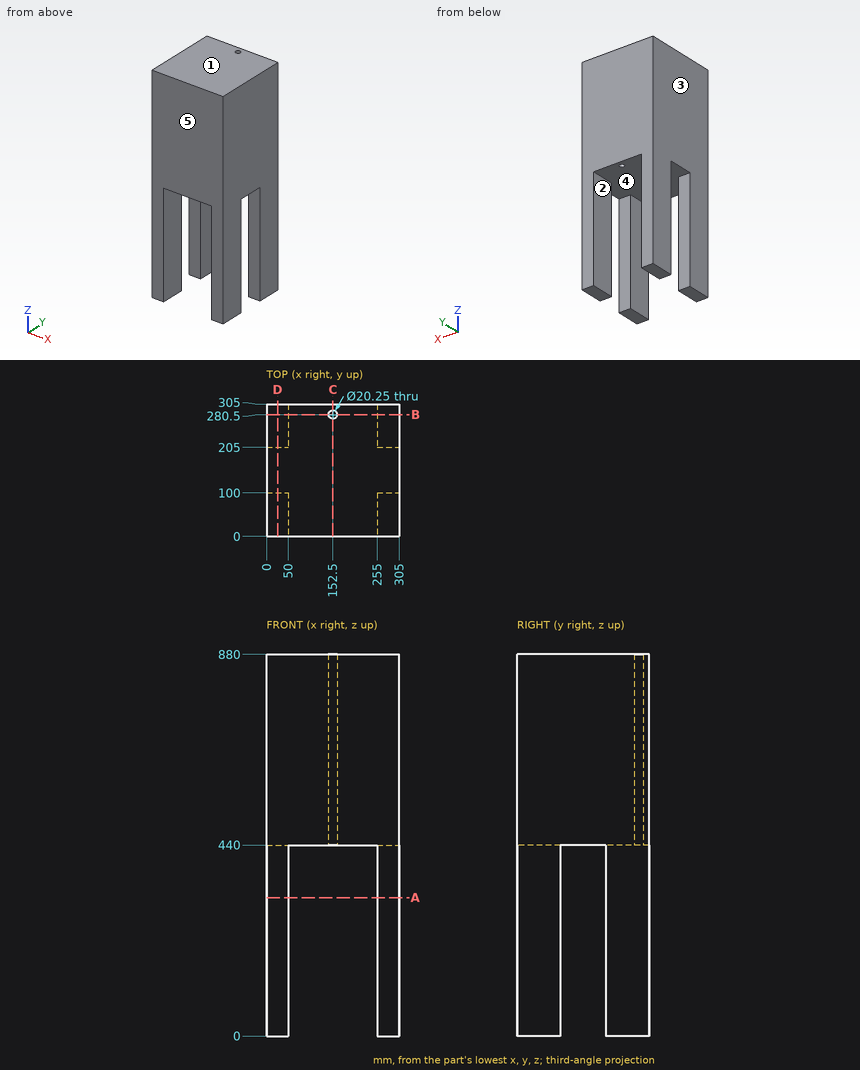
Could you check a few things on this drawing? It's one solid part, dimensions in mm from its lowest x, y, z. A direction names the side the tool comes from. Coordinates: 2 decimals unless noted, no trailing zeros. Order: outer loops, then holes, each group sorted by start corner. A loop starts at its lowest first (then second) coordinate and runs counter-clockwise, first axis right, second up.
1. If we section it at D-D (x = 25): Please give me the cut outline in (y, z), then the cut area to 3 significant figures.
2. I'm going to push a flat-ended pin straight in: pin 1 (1.5 mm diameter, centred on x = 136.5, y = 259.5, fed in from -Z). Where does the tip first touch, or does it pass through?
3. Thinking about a two-plate mould opening in Y: for the marked faces 3, 4 and 5, which applies, +Y half, -Y half, draft (parallel to the pull), parting line (faces both ways), or undercut?
4. I need wall thicknesses on line 1 (X direction, y = 280, z = 765); line 2 (Y direction, x = 152.5, z = 552.5) (3 decimals); line 3 (X direction, y = 248, z = 335). Which ranges of each line are inside material? Lowest first, please.
5. If we section it at B-B (y = 280.5): Please give me the cut outline in (x, z) (3 decimals).
6. If we section it at A-A (z = 319): Please give me the cut outline in (x, y).
7. For the marked faces 1 and 2, which set-ups out of +Z, -Z, +X, -X, +Y, -Y let a thin tool reach every point of the face, with its end or its side?
8. If we section it at C-C (x = 152.5): Please give me the cut outline in (y, z) (3 decimals).
Entries:
1. outline: (0, 0) - (100, 0) - (100, 440) - (205, 440) - (205, 0) - (305, 0) - (305, 880) - (0, 880) - close
1. area: 222,000 mm2
2. pin 1: stops at z = 440
3. face 3: draft
3. face 4: undercut
3. face 5: -Y half
4. line 1: x = 0 to 142.39, 162.61 to 305
4. line 2: y = 0 to 270.375, 290.625 to 305
4. line 3: x = 0 to 50, 255 to 305
5. outline: (0, 0) - (50, 0) - (50, 440) - (142.375, 440) - (142.375, 880) - (0, 880) - close; (162.625, 440) - (255, 440) - (255, 0) - (305, 0) - (305, 880) - (162.625, 880) - close
6. outline: (0, 0) - (50, 0) - (50, 100) - (0, 100) - close; (0, 205) - (50, 205) - (50, 305) - (0, 305) - close; (255, 0) - (305, 0) - (305, 100) - (255, 100) - close; (255, 205) - (305, 205) - (305, 305) - (255, 305) - close
7. face 1: +Z, +X, -X, +Y, -Y
7. face 2: -Z, +Y, -Y
8. outline: (0, 440) - (270.375, 440) - (270.375, 880) - (0, 880) - close; (290.625, 440) - (305, 440) - (305, 880) - (290.625, 880) - close
